from build123d import *

# Parameters (mm, degrees)
F0_W     = 38.1
F0_H     = 114.3
F3_DEPTH = 50.8
F2_W     = 38.1
F2_H     = 114.3
F4_DEPTH = 38.1
F1_W     = 38.1
F1_H     = 114.3
F5_DEPTH = 38.1
F6_D     = 12.7
F7_D     = 12.7
F8_D     = 12.7
F9_D     = 12.7
F10_R    = 5.08
F11_R    = 5.08
F12_R    = 5.08
F13_R    = 5.08


with BuildPart() as f3:
    # F0 (on Top) → F3 (new body)
    with BuildSketch(Plane.XY):
        Rectangle(F0_W, F0_H)
    extrude(amount=F3_DEPTH)

    # F2 (on Top) → F4 (join)
    with BuildSketch(Plane.XY):
        with Locations((38.1, 0)):
            Rectangle(F2_W, F2_H)
    extrude(amount=F4_DEPTH)

    # F1 (on Top) → F5 (join)
    with BuildSketch(Plane.XY):
        with Locations((-38.1, 0)):
            Rectangle(F1_W, F1_H)
    extrude(amount=F5_DEPTH)

    # F6 (through all)
    with Locations(Plane(origin=(0, 0, 0), x_dir=(1, 0, 0), z_dir=(0, 0, -1))):
        with Locations((37.4482907355, -32.3348678648)):
            Hole(F6_D / 2)

    # F7 (through all)
    with Locations(Plane(origin=(0, 0, 0), x_dir=(1, 0, 0), z_dir=(0, 0, -1))):
        with Locations((37.4482907355, 32.0340804756)):
            Hole(F7_D / 2)

    # F8 (through all)
    with Locations(Plane(origin=(0, 0, 0), x_dir=(1, 0, 0), z_dir=(0, 0, -1))):
        with Locations((-39.5538173616, -32.3348678648)):
            Hole(F8_D / 2)

    # F9 (through all)
    with Locations(Plane(origin=(0, 0, 0), x_dir=(1, 0, 0), z_dir=(0, 0, -1))):
        with Locations((-39.5538173616, 32.3348678648)):
            Hole(F9_D / 2)

    # F10
    f10_edges = [f3.edges().sort_by_distance(p)[0] for p in [
        (-57.15, -57.15, 19.05),
    ]]
    fillet(f10_edges, radius=F10_R)

    # F11
    f11_edges = [f3.edges().sort_by_distance(p)[0] for p in [
        (57.15, -57.15, 19.05),
    ]]
    fillet(f11_edges, radius=F11_R)

    # F12
    f12_edges = [f3.edges().sort_by_distance(p)[0] for p in [
        (57.15, 57.15, 19.05),
    ]]
    fillet(f12_edges, radius=F12_R)

    # F13
    f13_edges = [f3.edges().sort_by_distance(p)[0] for p in [
        (-57.15, 57.15, 19.05),
    ]]
    fillet(f13_edges, radius=F13_R)


solid = f3.part
Build history of the part. All positions in model axes, mm. A direction names the side the tool comes from. Give positions to 0.01 mm unless a question says otherwise; leave off trailing zeros. Loops run counter-clockwise (first coordinate to the right, second up) from the corner with the lowest first, then second, coordinate; pieces in that order, holes last. Notation, with made-up numbers: (33, 54.25) - (58, 54.25) arc R19 ccw to (58, 90.25) - close; hole circle Ø1 at (59.25, 66.25). An arc over 180 degrees is marked (long way). Write item = value, one per line. Start each with the question number.
1) Pull direction Y, two halves, no side cores. Call faces 4 (the cylindrical face through (55.622, -55.701, 19.317)), 5 (the cylindrical face through (42.129, -36.326, 19.317)), 6 (the flat face through (-1, 1, 0)): +Y half, -Y half, draft (parallel to the pull), parting line (faces both ways), or undercut.
2) Drop flat-ended pins along their axis: pin 1 Ø14 at (y, z) = (3.5, 46.5) entering from +X; pin 2 Ø20.5 at (x, y) = (-39.55, 32.33) entering from +Z. Give the stop position or say it passes through.
3) Band-saw the part on A-A on x = 39.5. Give the cut face in (y, z).
4) Band-saw the part on C-C on y = -35.5. Give the cut face in (x, z).
5) Probe probe 1 along Y at (x, z) = (37, 26); probe 2 along Y at (x, z) = (-45, 13.5); probe 3 along X at (y, z) = (14, 41). List the from-to ranges inside material, lowest first. Write a range as from..to.
6) Tool access for faces 1 (the flat face through (19.05, -1, 44)), 2 (the flat face through (-1, 57.15, 19)), 3 (the flat face through (-19.05, -1, 44)): list every direction of +Z, -Z, +X, -X, +Y, -Y with a clear straight run to the whole face (end or side of a thin tool).
7) Band-saw the part on D-D on z = 28. Give the cut face in (x, y).
8) Band-saw the part on B-B on y = -22.5. Give the cut face in (x, z).
Final values:
q1.face_4 = -Y half
q1.face_5 = undercut
q1.face_6 = draft
q2.pin_1 = 19.05
q2.pin_2 = 38.1
q3.outline = (-57.15, 0) - (-38.04, 0) - (-38.04, 38.1) - (-57.15, 38.1) - close; (-26.02, 0) - (26.33, 0) - (26.33, 38.1) - (-26.02, 38.1) - close; (38.34, 0) - (57.15, 0) - (57.15, 38.1) - (38.34, 38.1) - close
q4.outline = (-57.15, 0) - (-45.06, 0) - (-45.06, 38.1) - (-57.15, 38.1) - close; (-34.05, 0) - (32.13, 0) - (32.13, 38.1) - (19.05, 38.1) - (19.05, 50.8) - (-19.05, 50.8) - (-19.05, 38.1) - (-34.05, 38.1) - close; (42.77, 0) - (57.15, 0) - (57.15, 38.1) - (42.77, 38.1) - close
q5.probe_1 = -57.15..-38.37, -25.7..26, 38.67..57.15
q5.probe_2 = -57.15..-35.6, -29.07..29.07, 35.6..57.15
q5.probe_3 = -19.05..19.05
q6.face_1 = +Z, +X, +Y, -Y
q6.face_2 = +Z, -Z, +X, -X, +Y
q6.face_3 = +Z, -X, +Y, -Y
q7.outline = (-57.15, -52.07) arc R5.08 ccw to (-52.07, -57.15) - (52.07, -57.15) arc R5.08 ccw to (57.15, -52.07) - (57.15, 52.07) arc R5.08 ccw to (52.07, 57.15) - (-52.07, 57.15) arc R5.08 ccw to (-57.15, 52.07) - close; hole circle Ø12.7 at (-39.55, -32.33); hole circle Ø12.7 at (-39.55, 32.33); hole circle Ø12.7 at (37.45, -32.03); hole circle Ø12.7 at (37.45, 32.33)
q8.outline = (-57.15, 0) - (57.15, 0) - (57.15, 38.1) - (19.05, 38.1) - (19.05, 50.8) - (-19.05, 50.8) - (-19.05, 38.1) - (-57.15, 38.1) - close
